Part print with two shaded views. Sizes in mm from the minimum x, y, z corner. Give positions to 0.01 mm unless a question says otherwise; leave off trailing zeros. Write each loop counter-clockwise with the first axis right and the second up, starting at its lowest first coordinate (ties: lowest second). Pieces come first, ordered by that corner, then holes.
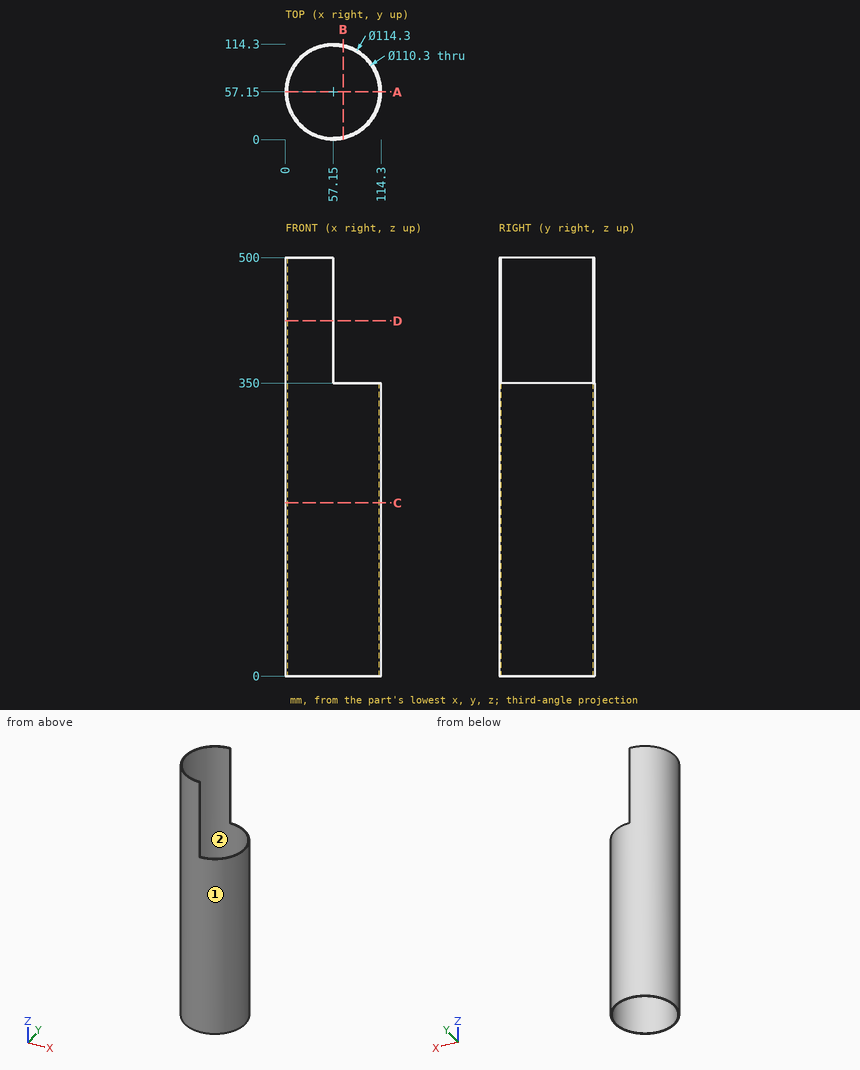
1) Saw through at A-A (y = 57.15). Write the cut outline in (x, z).
Check result:
outline: (0, 0) - (2, 0) - (2, 500) - (0, 500) - close; (112.3, 0) - (114.3, 0) - (114.3, 350) - (112.3, 350) - close
2) Mould opens along X. For the marked faces 1 and 2 say: +X half, -X half, draft (parallel to the pull), parting line (faces both ways), or undercut.
Check result:
face 1: parting line
face 2: undercut
3) Drill centre lines: L1, parallel to X at y = 57, z = 129; L2, parallel to X at y = 60, z = 224.5. Where is each one in solid material? Low to high.
Check result:
L1: x = 0 to 2, 112.3 to 114.3
L2: x = 0.07 to 2.07, 112.23 to 114.23
4) Flat gauge pins, fed straight in: P1, Ø10, axis at y = 18, z = 298, coming from the +X side; P2, Ø1.5, axis at x = 29, z = 238, coming from the +Y side; P3, Ø4, axis at x = 95.5, z = 201.5, coming from the +Y side. Where does each tip first touch, or does it go through?
Check result:
P1: stops at x = 102.97
P2: stops at y = 107.3
P3: stops at y = 101.25
5) Saw through at D-D (z = 424.5). Write the cut outline in (x, y).
Check result:
outline: (57.15, 0) - (57.15, 2) arc R55.15 cw to (57.15, 112.3) - (57.15, 114.3) arc R57.15 ccw to start
6) Saw through at C-C (z = 207). Write the cut outline in (x, y), and give its area (3 significant figures).
Check result:
outline: circle Ø114.3 at (57.15, 57.15); hole circle Ø110.3 at (57.15, 57.15)
area: 706 mm2
7) Saw through at B-B (x = 69). Write the cut outline in (y, z), and give its area (3 significant figures).
Check result:
outline: (1.24, 0) - (3.29, 0) - (3.29, 350) - (1.24, 350) - close; (111.01, 0) - (113.06, 0) - (113.06, 350) - (111.01, 350) - close
area: 1,430 mm2
